Can you work these out from the model? Positions are in its coordinate system, mm. A direction names the side the tool comes from. Give positions to 0.01 mm unless a question says otherwise; leave off trailing zeros. Loops run counter-clockwise (first coordinate to the right, second up) from the corner with the lowest first, then second, coordinate; pieces in that order, holes last. Notation, with made-up numbers: (83.5, -32.75) - (95.5, -32.75) arc R29 cw to (95.5, 5.25) - close; hole circle Ø8 at (27, -19). An arc over 180 degrees is marked (long way). Write item = value, one per line.
Autodesk Inventor part; units mm, degrees
ref_plane "YZ Plane" through (0, 0, 0) normal (1, 0, 0) x (0, 1, 0)
ref_plane "XZ Plane" through (0, 0, 0) normal (0, 1, 0) x (-1, 0, 0)
ref_plane "XY Plane" through (0, 0, 0) normal (0, 0, 1) x (1, 0, 0)
sketch "Sketch1" plane through (0, 0, 0) normal (0, 0, 1) x (1, 0, 0)
  line L0 (0, 0) -> (47.25, 0)
  line L1 (47.25, 0) -> (47.25, -4)
  line L2 (47.25, -4) -> (50, -4)
  line L3 (50, -4) -> (50, 65)
  line L4 (50, 65) -> (0, 65)
  line L5 (0, 65) -> (0, 0)
  dimension "d0" = 100
  dimension "d1" = 94.5
  dimension "d2" = 4
  dimension "d3" = 65
revolve "Revolution1" add sketch "Sketch1" angle 360 about axis through (0, 65, 0) along (0, -1, 0)
sketch "Sketch2" plane through (0, 0, 0) normal (0, 0, 1) x (1, 0, 0)
  line L0 (-50, 65) -> (-50, -4)
  line L1 (-50, 12) -> (50, 12)
  circle A0 centre (0, 40) radius 25
  line L2 (-50, 65) -> (50, 65)
  line L3 (0, 0) -> (0, 65) construction
  arc A1 (-50, 12) -> (-24.9999, 40.0686) centre (-53.3441, 40.1463) ccw
  arc A2 (24.9999, 40.0686) -> (50, 12) centre (53.3441, 40.1463) ccw
  line L4 (50, 65) -> (50, -4)
  point P0 (0, 12)
  point P1 (0, 65)
  dimension "d5" = 12
  dimension "d6" = 50
  dimension "d7" = 28.0686
  dimension "d8" = 28.0686
extrude "Extrusion1" cut sketch "Sketch2" along normal through all both and the other way through all contours L2 A0 A1 L0 | L2 L4 A2 A0
sketch "Sketch4" plane through (0, 0, 0) normal (1, 0, 0) x (0, 1, 0)
  line L0 (65, 50) -> (-4, 50)
  line L1 (12, 50) -> (12, 50)
  line L2 (14, -48) -> (65, -48)
  line L3 (14, 48) -> (65, 48)
  line L4 (65, 50) -> (65, -50)
  line L5 (0, 47.25) -> (0, -47.25)
  line L6 (65, -50) -> (-4, -50)
  arc A0 (12, 50) -> (14, 48) centre (14, 50) ccw
  line L7 (12, -50) -> (12, -50)
  arc A1 (14, -48) -> (12, -50) centre (14, -50) ccw
  line L8 (65, -39) -> (12, -39)
  line L9 (12, -39) -> (12, 39)
  line L10 (12, 39) -> (65, 39)
  line L11 (65, 39) -> (65, -39)
  line L12 (12, -50) -> (65, -50)
  line L13 (65, -48) -> (65, -50)
  line L14 (12, 50) -> (65, 50)
  line L15 (65, 50) -> (65, 48)
  point P0 (0, 0)
  point P1 (12, -48)
  point P2 (65, 39)
  dimension "d14" = 2
  dimension "d15" = 12
  dimension "d16" = 2
  dimension "d17" = 2
  dimension "d18" = 2
  dimension "d19" = 12
  dimension "d20" = 9
  dimension "d21" = 9
extrude "Extrusion2" cut sketch "Sketch4" along normal through all both and the other way through all
sketch "Sketch5" plane through (0, 40, 48) normal (0, 0, 1) x (1, 0, 0)
  line L0 (-31.289, -28) -> (31.289, -28)
  line L1 (-31.289, -28) -> (-25.0769, -28)
  spline S0 degree 7 poles (-24.9999, 0.0686) (-25.0047, -1.665) (-25.1331, -3.4008) (-25.3859, -5.1281) (-25.7625, -6.8362) (-26.2611, -8.5141) (-26.8789, -10.1513) (-27.8149, -12.1783) (-28.0274, -12.6153) (-28.2486, -13.0478) (-28.478, -13.4752) (-28.7156, -13.8974) (-28.961, -14.3139) (-29.4863, -15.1662) (-29.7674, -15.6012) (-30.057, -16.029) (-30.3544, -16.4489) (-30.6593, -16.8605) (-30.971, -17.2634) (-31.289, -17.6573) knots 0 0 0 0 0 0 0 0 0.63383 0.63383 0.63383 0.63383 0.63383 0.63383 0.810222 0.810222 0.810222 0.810222 0.810222 0.810222 1 1 1 1 1 1 1 1
  line L2 (-31.289, -17.6573) -> (-31.289, -28)
  spline S1 degree 7 poles (31.289, -17.6573) (30.9729, -17.2657) (30.6629, -16.8652) (30.3597, -16.456) (30.0639, -16.0387) (29.7758, -15.6136) (29.4961, -15.1814) (28.9731, -14.3341) (28.7285, -13.9199) (28.4918, -13.5001) (28.263, -13.075) (28.0425, -12.645) (27.8305, -12.2104) (26.8905, -10.182) (26.269, -8.5404) (25.7672, -6.8576) (25.3883, -5.1443) (25.1339, -3.4117) (25.0047, -1.6704) (24.9999, 0.0686) knots 0 0 0 0 0 0 0 0 0.188676 0.188676 0.188676 0.188676 0.188676 0.188676 0.364186 0.364186 0.364186 0.364186 0.364186 0.364186 1 1 1 1 1 1 1 1
  line L3 (31.289, -28) -> (31.289, -17.6573)
  arc A0 (24.9999, 0.0686) -> (31.289, -17.6573) centre (53.3441, 0.1463) ccw
  line L4 (24.9999, 0.0686) -> (25.0769, -28)
  line L5 (25.0769, -28) -> (31.289, -28)
  arc A1 (-31.289, -17.6573) -> (-24.9999, 0.0686) centre (-53.3441, 0.1463) ccw
  line L6 (-24.9999, 0.0686) -> (-25.0769, -28)
  point P0 (0, -40)
  point P1 (24.9999, -28)
extrude "Extrusion3" cut sketch "Sketch5" along normal through all both and the other way through all
sketch "Sketch6" plane through (0, 40, -39) normal (0, 0, 1) x (1, 0, 0)
  arc A0 (14, 20.7123) -> (-14, 20.7123) centre (0, 0) ccw
  circle A1 centre (0, 0) radius 10
  point P0 (0, -40)
  dimension "d26" = 20
extrude "Extrusion4" cut sketch "Sketch6" along normal blind 83 and the other way blind 5
equation "\"d8\" = d7"
equation "\"d21\" = d20"
properties part number "Arm 1 v0.1"
Q1. Which directions (+Z, -Z, +X, -X, +Y, -Y) give clear straight access to the entire face, cutting with the end or side of a thin tool? Please do faces 4 (the flat face through (0, 26, 39)), 5 (the flat face through (-1, 0, 1)), 6 (the cylindrical face through (-2.17, 30.24, -41.46)), 7 (the flat face through (0, 39, 48)).
Output:
face_4 = +X, -X, +Y
face_5 = -Y
face_6 = none
face_7 = +Z, +X, -X, +Y
Q2. We'd pull the mould along Y, two halves only. Please class faces 1 (the flat face through (0, 40, -44)), 2 (the flat face through (0, 27, -39)), 3 (the flat face through (-1, 12, -1)): released by +Y, released by -Y, zero draft, split by the parting line, or undercut.
Output:
face_1 = undercut
face_2 = zero draft
face_3 = released by +Y
Q3. Imagine slicing it at D-D, the plane y = 32. Write out the boundary of the cut face in (x, z).
Output:
outline = (-25.02, -43.29) arc R50 ccw to (-14, -48) - (14, -48) arc R50 ccw to (25.02, -43.29) - (25.02, -39) - (6, -39) - (6, -44) - (-6, -44) - (-6, -39) - (-25.02, -39) - close; (-25.02, 39) - (-6, 39) - (-6, 44) - (6, 44) - (6, 39) - (25.02, 39) - (25.02, 43.29) arc R50 ccw to (14, 48) - (-14, 48) arc R50 ccw to (-25.02, 43.29) - close
Q4. Imagine slicing it at A-A, the plane x = 0. Write out the boundary of the cut face in (y, z).
Output:
outline = (-4, -50) - (12, -50) arc R2 cw to (14, -48) - (65, -48) - (65, -39) - (50, -39) - (50, -44) - (30, -44) - (30, -39) - (12, -39) - (12, 39) - (30, 39) - (30, 44) - (50, 44) - (50, 39) - (65, 39) - (65, 48) - (14, 48) arc R2 cw to (12, 50) - (-4, 50) - (-4, 47.25) - (0, 47.25) - (0, -47.25) - (-4, -47.25) - close
Q5. Imagine slicing it at B-B, the plane y = 20.5. Write out the boundary of the cut face in (x, z), then the cut area to 3 significant figures.
Output:
outline = (-25.05, -43.27) arc R50 ccw to (-14, -48) - (14, -48) arc R50 ccw to (25.05, -43.27) - (25.05, -39) - (-25.05, -39) - close; (-25.05, 39) - (25.05, 39) - (25.05, 43.27) arc R50 ccw to (14, 48) - (-14, 48) arc R50 ccw to (-25.05, 43.27) - close
area = 809 mm2
Q6. Imagine slicing it at C-C, the plane z = 0. Write out the boundary of the cut face in (x, y).
Output:
outline = (-50, -4) - (-47.25, -4) - (-47.25, 0) - (47.25, 0) - (47.25, -4) - (50, -4) - (50, 12) - (-50, 12) - close
Q7. For pin 1 (3 mm diameter, centred on x = -19, z = 31.5, fed in from -Y); pin 2 (1 mm diameter, centred on x = -35.5, z = 38.5, fed in from +Y); pin 3 (16 mm diameter, centred on x = 3.5, y = 45, fed in from -Z); pin 4 (1 mm diameter, centred on x = 7.5, y = 39, fed in from +Z), each with a flat end and sliding along its axis, tell me the tip position at first contact or that it passes through.
Output:
pin_1 = 0
pin_2 = through
pin_3 = -48
pin_4 = 48
Q8. I need wall thicknesses on L1, parallel to Y at x = 0, z = -41.4; L2, parallel to X at y = 40, z = 42; L3, parallel to Z at x = -4, y = 59. Which ranges of each line are inside material? Lowest first, please.
Output:
L1 = 0 to 30, 50 to 65
L2 = -25 to -10, 10 to 25
L3 = -48 to -39, 39 to 48
